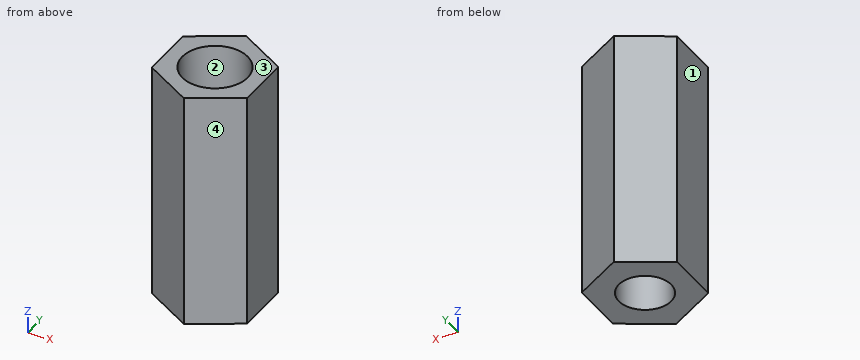
from build123d import *

# Parameters (mm, degrees)
F1_DEPTH = 40
F3_D     = 11
F3_DEPTH = 10
F3_TIP   = 3.3047334047
F4_D     = 8.8


with BuildPart() as f1:
    # F0 (on Top) → F1 (new body)
    with BuildSketch(Plane.XY):
        Polygon((8, -4.6188021535), (8, 4.6188021535), (0, 9.237604307), (-8, 4.6188021535), (-8, -4.6188021535), (0, -9.237604307), align=None)
    extrude(amount=F1_DEPTH)

    # F3
    with Locations(Plane.XY.offset(40)):
        with Locations((0, 0)):
            Hole(F3_D / 2, depth=F3_DEPTH)
            with Locations((0, 0, -(F3_DEPTH + F3_TIP / 2))):  # 118° drill point
                Cone(0, F3_D / 2, F3_TIP, mode=Mode.SUBTRACT)

    # F4 (through all)
    with Locations(Plane.XY.offset(40)):
        with Locations((0, 0)):
            Hole(F4_D / 2)


solid = f1.part
Source: CAD feature listing. Evaluate the final solid. Frame: model axes, mm. Face numbers are marked on the shaded views. Coordinates: 2 decimals unless noted, no trailing zeros. Write each loop counter-clockwise with the first axis right and the second up, starting at its lowest first coordinate (ties: lowest second). Pieces come first, ordered by that corner, then holes. Notation, with made-up numbers: M -18,23.25 L 16,23.25 A22 ccw 16,62.25 Z; hole C 58.5,35 d2. An arc over 180 degrees is marked long. Use a Markdown table: item, result.
1) Mould query, pull axis X, two halves, no side actions, for the marked faces 1, 2, 3 and 4. Classes: pulls with the +X half, pulls with the -X half, needs draft (parallel to the pull), parting line crosses it, or undercut.
Conclusion:
| item | result |
|---|---|
| face 1 | pulls with the -X half |
| face 2 | undercut |
| face 3 | needs draft |
| face 4 | pulls with the +X half |
2) First-contact query: pin 1 Ø8 at (y, z) = (-5.5, 21.5) entering from +X; pin 2 Ø5 at (x, z) = (-0.5, 35) entering from -Y. Flat tips, straight axial feed; report the tip coordinate or a pass-through.
Conclusion:
| item | result |
|---|---|
| pin 1 | stops at x = 8 |
| pin 2 | stops at y = -9.24 |
3) Ray query, L1, parallel to X at y = 0, z = 14.75; L2, parallel to X at y = 0, z = 34; L3, parallel to Y at x = 0, z = 34.5. Return the intervals inside material, ascending.
Conclusion:
| item | result |
|---|---|
| L1 | x = -8 to -4.4, 4.4 to 8 |
| L2 | x = -8 to -5.5, 5.5 to 8 |
| L3 | y = -9.24 to -5.5, 5.5 to 9.24 |
4) Section B-B, the plane z = 9. Output: boundary loops of the cut face in (x, y).
Conclusion:
| item | result |
|---|---|
| outline | M -8,-4.62 L 0,-9.24 L 8,-4.62 L 8,4.62 L 0,9.24 L -8,4.62 Z; hole C 0,0 d8.8 |
5) Section C-C, the plane z = 30.5. Output: boundary loops of the cut face in (x, y), then the cut area to 3 significant figures.
Conclusion:
| item | result |
|---|---|
| outline | M -8,-4.62 L 0,-9.24 L 8,-4.62 L 8,4.62 L 0,9.24 L -8,4.62 Z; hole C 0,0 d11 |
| area | 127 mm^2 |
6) Section A-A, the plane y = 0. Output: boundary loops of the cut face in (x, z), then the cut area to 3 significant figures.
Conclusion:
| item | result |
|---|---|
| outline | M -8,0 L -4.4,0 L -4.4,29.34 L -5.5,30 L -5.5,40 L -8,40 Z; M 4.4,0 L 8,0 L 8,40 L 5.5,40 L 5.5,30 L 4.4,29.34 Z |
| area | 265 mm^2 |
